Geometry: see drawing. Coordinates: mm, zero at the bounding-box minimum. A direction names the side the tool comes from. Round coordinates to 2 decimals unless told otherwise and drop trailing zeros. Write each loop counter-clockwise with the first axis right and the second up, starting at its lowest first coordinate (ties: lowest second). Pieces come first, ordered by that corner, then holes. Notation, with made-up numbers: (71.5, 7.25) - (85.5, 7.25) arc R29 cw to (85.5, 28.25) - close; hole circle Ø11 at (69.5, -15). An arc over 180 degrees is marked (long way). Use a Markdown table: item, result. Add a question column.
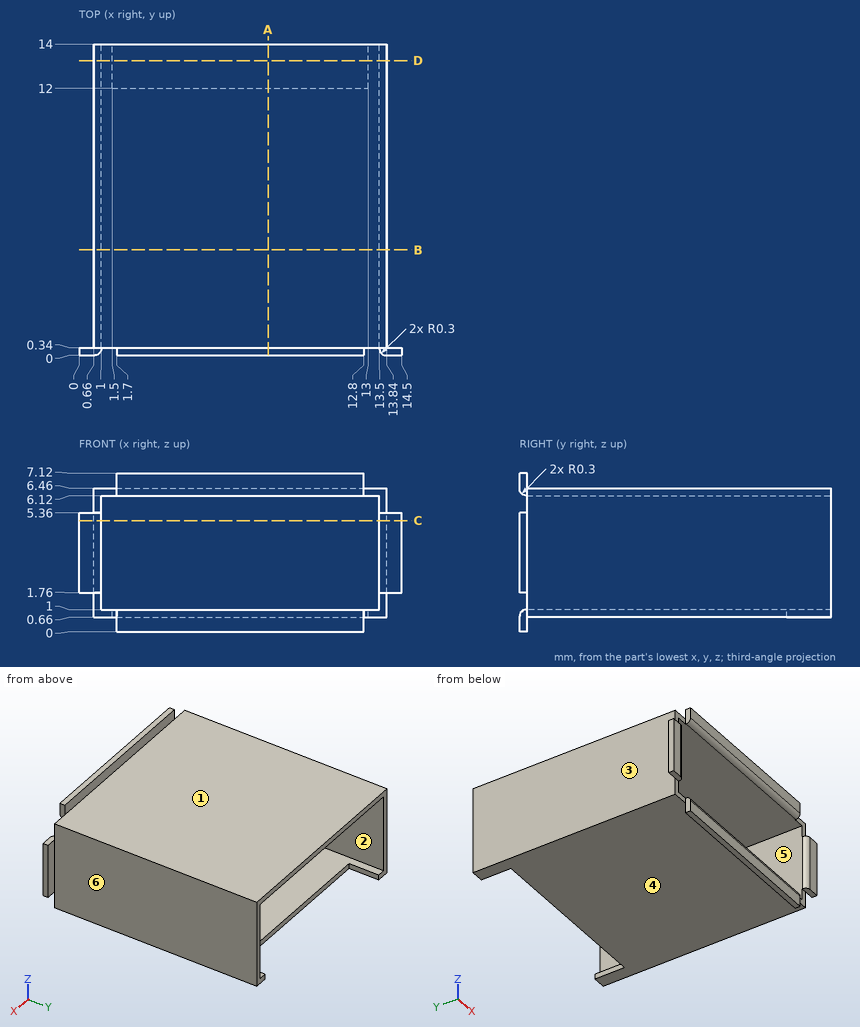
1) Section A-A, the plane x = 8.5. Return the cut outline in (y, z), then the cut area to 3 significant figures.
2) Section C-C, the plane z = 5. Return the cut outline in (x, y), then the cut area to 3 significant figures.
3) Material intervals for L1, parallel to X at y = 8, z = 5.75; L2, parallel to Z at x = 8.5, y = 5.75; L3, parallel to Y at x = 8, z = 6.75, sorted ascending. Write a range as from..to.
4) Section B-B, the plane y = 4.75. Return the cut outline in (x, z), then the cut area to 3 significant figures.
5) Section D-D, the plane y = 13.25. Return the cut outline in (x, z), then the cut area to 3 significant figures.
6) Set-up query: the marked faces 1, 2 and 3. Return all of +Z, -Z, +X, -X, +Y, -Y with unobstructed straight access to the full face (end or side cutting, diameter ignored); none if empty.
7) Pin query (flat end, axial travel): P1, Ø6, axis at x = 3, y = 10.5, coming from the +Z side; P2, Ø1.5, axis at y = 4.5, z = 2.5, coming from the -X side; P3, Ø2, axis at x = 2.5, y = 4.5, coming from the -Z side. Return the tip coordinate at first contact, or that it passes through.
8) Draft query along X for the marked faces 4, 5 and 6. Return one class per face: released by +X, released by -X, zero draft, split by the parting line, or undercut.
Output values:
| question | item | result |
|---|---|---|
| 1 | outline | (0, 0) - (0.34, 0) - (0.34, 0.66) - (12, 0.66) - (12, 1) - (0.3, 1) arc R0.3 ccw to (0, 0.7) - close; (0, 6.42) arc R0.3 ccw to (0.3, 6.12) - (14, 6.12) - (14, 6.46) - (0.34, 6.46) - (0.34, 7.12) - (0, 7.12) - close |
| 1 | area | 9.25 mm^2 |
| 2 | outline | (0, 0) - (0.7, 0) arc R0.3 ccw to (1, 0.3) - (1, 14) - (0.66, 14) - (0.66, 0.34) - (0, 0.34) - close; (13.5, 0.3) arc R0.3 ccw to (13.8, 0) - (14.5, 0) - (14.5, 0.34) - (13.84, 0.34) - (13.84, 14) - (13.5, 14) - close |
| 2 | area | 9.93 mm^2 |
| 3 | L1 | x = 0.66..1, 13.5..13.84 |
| 3 | L2 | z = 0.66..1, 6.12..6.46 |
| 3 | L3 | y = 0..0.34 |
| 4 | outline | (0.66, 0.66) - (13.84, 0.66) - (13.84, 6.46) - (0.66, 6.46) - close; hole (1, 1) - (13.5, 1) - (13.5, 6.12) - (1, 6.12) - close |
| 4 | area | 12.4 mm^2 |
| 5 | outline | (0.66, 0.66) - (1.5, 0.66) - (1.5, 1) - (1, 1) - (1, 6.12) - (13.5, 6.12) - (13.5, 1) - (13, 1) - (13, 0.66) - (13.84, 0.66) - (13.84, 6.46) - (0.66, 6.46) - close |
| 5 | area | 8.53 mm^2 |
| 6 | face 1 | +Z, +X, -X, +Y |
| 6 | face 2 | +Y, -Y |
| 6 | face 3 | +Z, -Z, -X, +Y |
| 7 | P1 | stops at z = 6.46 |
| 7 | P2 | stops at x = 0.66 |
| 7 | P3 | stops at z = 0.66 |
| 8 | face 4 | zero draft |
| 8 | face 5 | undercut |
| 8 | face 6 | released by +X |
